from build123d import *

# Parameters (mm, degrees)
F0_R     = 1.49987
F1_DEPTH = 1.89738


with BuildPart() as f1:
    # F0 (on Front) → F1 (new body)
    with BuildSketch(Plane.XZ):
        with BuildLine():
            Line((-35.355524, 44.232099), (-41.705524, 44.232099))
            Line((-41.705524, 44.232099), (-41.705524, 42.644599))
            Line((-41.705524, 42.644599), (-54.405524, 42.644599))
            Line((-54.405524, 42.644599), (-54.405524, 44.232099))
            Line((-54.405524, 44.232099), (-60.755524, 44.231093))
            Line((-60.755524, 44.231093), (-60.755524, 44.224526))
            ThreePointArc((-60.755524, 44.224526), (-63.922951, 41.057099), (-60.755524, 37.889672))
            Line((-60.755524, 37.889672), (-60.755524, 37.883105))
            Line((-60.755524, 37.883105), (-54.405524, 37.882099))
            Line((-54.405524, 37.882099), (-54.405524, 39.469599))
            Line((-54.405524, 39.469599), (-41.705524, 39.469599))
            Line((-41.705524, 39.469599), (-41.705524, 37.882099))
            Line((-41.705524, 37.882099), (-35.355524, 37.882099))
            Line((-35.355524, 37.882099), (-35.355524, 37.883105))
            ThreePointArc((-35.355524, 37.883105), (-32.18153, 41.057099), (-35.355524, 44.231093))
            Line((-35.355524, 44.231093), (-35.355524, 44.232099))
        make_face()
        with Locations((-60.755524, 41.057099)):
            Circle(F0_R, mode=Mode.SUBTRACT)
        with Locations((-35.355524, 41.057099)):
            Circle(F0_R, mode=Mode.SUBTRACT)
    extrude(amount=F1_DEPTH)


solid = f1.part
The model under review builds one solid part; all positions refer to its coordinate system, in mm. A direction names the side the tool comes from. Round coordinates to 2 decimals unless told otherwise and drop trailing zeros. Write each loop counter-clockwise with the first axis right and the second up, starting at its lowest first coordinate (ties: lowest second). Pieces come first, ordered by that corner, then holes. Notation, with made-up numbers: M 19,29 L 61,29 A29 ccw 61,65 Z; hole C 82.5,9.5 d5. An arc over 180 degrees is marked long. Use a Markdown table: item, result. Add a question column.
Q1. Machinability: for faces 1 (the face through (-48, -1, 42.645)), 2 (the face through (-48, -1, 39.47)), 3 (the face through (-33.925, -0.935, 41.508)), which of the approach directions +Z, -Z, +X, -X, +Y, -Y give a long, thin tool a straight path to every point of the face, cutting with its end or side? Answer none if there is none.
Q2. We need section A-A, the plane z = 39. State the section outline as (x, y) points, plus the area to 3 significant figures.
Q3. To check wall thickness, follow line 1 (X direction, y = -1.65, z = 41); line 2 (X direction, y = -0.2, z = 40); line 3 (Z direction, x = -44.5, y = -1.75). State the ranges of each line that lie inside material, in increasing order.
Q4. The part is to be moulded in two halves that separate along X. For faces 4 (the face through (-41.706, -1, 39)), 5 (the face through (-48, -1.897, 41)), 6 (the face through (-32.182, -0.935, 40.987)), say which applies: pulls with the +X half, pulls with the -X half, needs draft (parallel to the pull), parting line crosses it, or undercut.
Q5. We need section C-C, the plane z = 40.25. State the section outline as (x, y) points.
Q6. Insertion check: pin 1 (0.5 mm diameter, centred on y = -1.5, z = 43, fed in from +X); pin 2 (0.5 mm diameter, centred on y = -1, z = 38.5, fed in from -X); pin 3 (0.6 mm diameter, centred on x = -50.5, y = -1, fed in from +Z). Each pin has a flat end and moves straight along its axis. Give the tip position at first contact, or say it passes through.
Q7. We need section B-B, the plane x = -36.5. State the section outline as (y, z) points, plus the area to 3 significant figures.
Q8. We need section D-D, the plane y = -0.35. Count the separate pieces of the cut face and the enclosed holes in it, plus the area to 3 significant figures.
Findings below:
| question | item | result |
|---|---|---|
| 1 | face 1 | +Z, +Y, -Y |
| 1 | face 2 | -Z, +Y, -Y |
| 1 | face 3 | +Y, -Y |
| 2 | outline | M -63.16,-1.9 L -54.41,-1.9 L -54.41,0 L -63.16,0 Z; M -41.71,-1.9 L -32.94,-1.9 L -32.94,0 L -41.71,0 Z |
| 2 | area | 33.3 mm² |
| 3 | line 1 | x = -63.92 to -62.25, -59.26 to -36.85, -33.86 to -32.18 |
| 3 | line 2 | x = -63.74 to -61.82, -59.69 to -36.42, -34.29 to -32.36 |
| 3 | line 3 | z = 39.47 to 42.64 |
| 4 | face 4 | undercut |
| 4 | face 5 | needs draft |
| 4 | face 6 | pulls with the +X half |
| 5 | outline | M -63.82,-1.9 L -62.02,-1.9 L -62.02,0 L -63.82,0 Z; M -59.49,-1.9 L -36.62,-1.9 L -36.62,0 L -59.49,0 Z; M -34.09,-1.9 L -32.29,-1.9 L -32.29,0 L -34.09,0 Z |
| 6 | pin 1 | stops at x = -32.67 |
| 6 | pin 2 | stops at x = -62.93 |
| 6 | pin 3 | stops at z = 42.64 |
| 7 | outline | M -1.9,37.88 L 0,37.88 L 0,40.09 L -1.9,40.09 Z; M -1.9,42.03 L 0,42.03 L 0,44.23 L -1.9,44.23 Z |
| 7 | area | 8.37 mm² |
| 8 | separate pieces | 1 |
| 8 | enclosed holes | 2 |
| 8 | area | 138 mm² |
